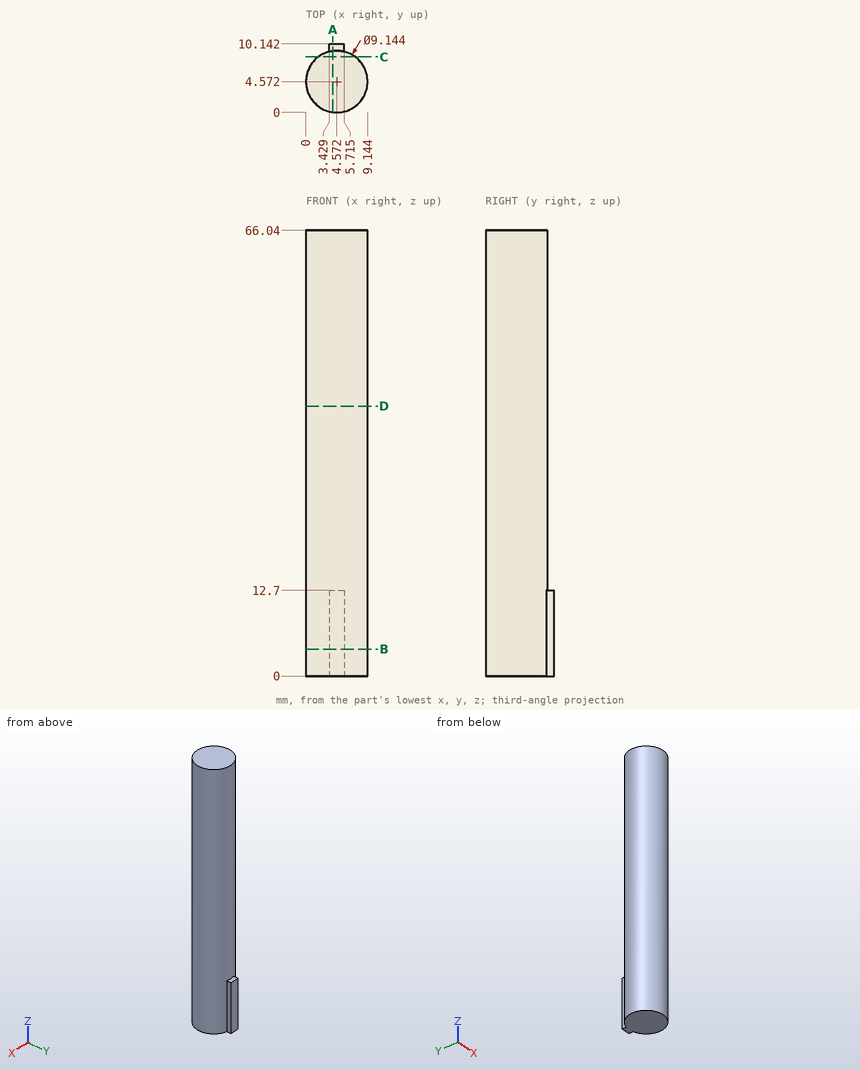
Job drawing, mm, ordinate dimensions from the low corner. One solid piece. Coordinates: 2 decimals unless noted, no trailing zeros. Order: outer loops, then holes, each group sorted by start corner. A loop starts at its lowest first (then second) coordinate and runs counter-clockwise, first axis right, second up. Notation, with made-up numbers: (16, 27) -> (47, 27) arc R7 cw to (47, 40) -> close; hole circle Ø9 at (46.25, 78). An arc over 180 degrees is marked (long way). Answer in a Markdown table with one row per item. Add a question column.
Q1. Band-saw the part on A-A, the plane x = 4. List the corners of the cut face in (y, z), then the cut area to 3 significant figures.
Q2. Band-saw the part on D-D, the plane z = 40. List the corners of the cut face in (x, y).
Q3. Drop flat-ended pins along their axis: pin 1 (1.5 mm diameter, centred on y = 3.5, z = 39, fed in from -X); pin 2 (5 mm diameter, centred on y = 9, z = 8.5, fed in from -X); pin 3 (1.5 mm diameter, centred on y = 3.5, z = 28.5, fed in from +X). Give the stop position or say it passes through.
Q4. Wall check: line 1 along X through (y, z) = (4.75, 63.5); line 2 along X through (y, z) = (7, 45.5); line 3 along Y through (x, z) = (8.5, 63.5). Give the ranges that are in metal, low to high. Write a range as [from, to].
Q5. Band-saw the part on B-B, the plane z = 4. List the corners of the cut face in (x, y) (1 decimal).
Q6. Band-saw the part on C-C, the plane y = 8.25. List the corners of the cut face in (x, z).
Answers follow:
| question | item | result |
|---|---|---|
| 1 | outline | (0.04, 0) -> (10.14, 0) -> (10.14, 12.7) -> (9.11, 12.7) -> (9.11, 66.04) -> (0.04, 66.04) -> close |
| 1 | area | 612 mm^2 |
| 2 | outline | circle Ø9.14 at (4.57, 4.57) |
| 3 | pin 1 | x = 0.01 |
| 3 | pin 2 | x = 0.43 |
| 3 | pin 3 | x = 9.13 |
| 4 | line 1 | [0, 9.14] |
| 4 | line 2 | [0.7, 8.45] |
| 4 | line 3 | [2.23, 6.91] |
| 5 | outline | (3.4, 9) arc R4.6 ccw (long way) to (5.7, 9) -> (5.7, 10.1) -> (3.4, 10.1) -> close |
| 6 | outline | (1.86, 0) -> (7.29, 0) -> (7.29, 66.04) -> (1.86, 66.04) -> close |
